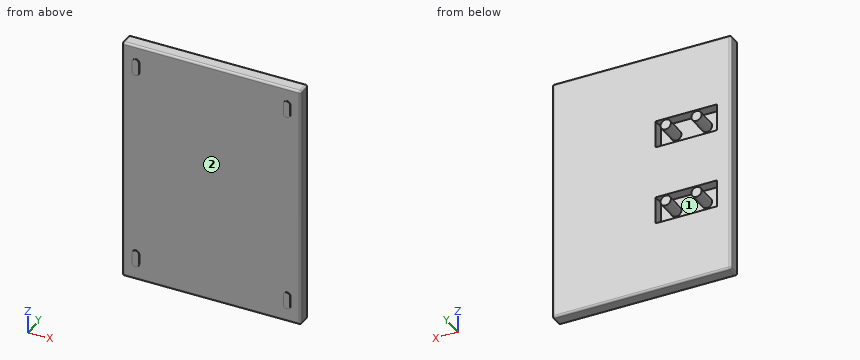
Autodesk Inventor part; units mm, degrees
ref_plane "YZ Plane" through (0, 0, 0) normal (1, 0, 0) x (0, 1, 0)
ref_plane "XZ Plane" through (0, 0, 0) normal (0, 1, 0) x (-1, 0, 0)
ref_plane "XY Plane" through (0, 0, 0) normal (0, 0, 1) x (1, 0, 0)
sketch "Sketch1" plane through (0, 0, 0) normal (0, 1, 0) x (-1, 0, 0)
  line L0 (0, 0) -> (260, 0)
  line L1 (260, 0) -> (260, -360)
  line L2 (260, -360) -> (0, -360)
  line L3 (0, -360) -> (0, 0)
  line L4 (240, -101.4) -> (150.6, -101.4)
  line L5 (150.6, -101.4) -> (150.6, -141.4)
  line L6 (150.6, -141.4) -> (240, -141.4)
  line L7 (240, -141.4) -> (240, -101.4)
  line L8 (240, -218.6) -> (150.6, -218.6)
  line L9 (150.6, -218.6) -> (150.6, -258.6)
  line L10 (150.6, -258.6) -> (240, -258.6)
  line L11 (240, -258.6) -> (240, -218.6)
  circle A0 centre (217.65, -121.4) radius 7.5
  circle A1 centre (172.95, -121.4) radius 7.5
  circle A2 centre (217.65, -238.6) radius 7.5
  circle A3 centre (172.95, -238.6) radius 7.5
  point P0 (240, -121.4)
  point P1 (150.6, -238.6)
  point P2 (240, -238.6)
  dimension "d0" = 260
  dimension "d1" = 360
  dimension "d2" = 89.4
  dimension "d3" = 40
  dimension "d4" = 89.4
  dimension "d5" = 40
  dimension "d8" = 15
  dimension "d9" = 15
  dimension "d11" = 22.35
  dimension "d12" = 15
  dimension "d13" = 15
  dimension "d14" = 22.35
  dimension "d15" = 22.35
  dimension "d16" = 22.35
  dimension "d17" = 20
  dimension "d61" = 117.2
  dimension "d62" = 101.4
  dimension "d63" = 101.4
extrude "Extrusion1" add sketch "Sketch1" along normal blind 20 contours L0 L1 L2 L3
extrude "Extrusion2" add sketch "Sketch1" along normal blind 5 contours L7 L6 L5 L4 | L11 L10 L9 L8
extrude "Extrusion3" add sketch "Sketch1" along normal blind 35 contours A0 | A1 | A2 | A3
sketch "Sketch2" plane through (0, 20, 0) normal (0, 1, 0) x (1, 0, 0)
  point P0 (0, 0)
sketch "Sketch4" plane through (0, 0, 0) normal (0, -1, 0) x (1, 0, 0)
  line L0 (-240, -335) -> (-240, -320) construction
  line L1 (-235, -335) -> (-235, -320)
  line L2 (-245, -320) -> (-245, -335)
  arc A0 (-245, -335) -> (-235, -335) centre (-240, -335) ccw
  arc A1 (-235, -320) -> (-245, -320) centre (-240, -320) ccw
  line L3 (-260, -360) -> (-260, 0)
  line L4 (0, -360) -> (-260, -360)
  line L5 (-240, -40) -> (-240, -25) construction
  line L6 (-235, -40) -> (-235, -25)
  line L7 (-245, -25) -> (-245, -40)
  arc A2 (-245, -40) -> (-235, -40) centre (-240, -40) ccw
  arc A3 (-235, -25) -> (-245, -25) centre (-240, -25) ccw
  line L8 (-20, -40) -> (-20, -25) construction
  line L9 (-15, -40) -> (-15, -25)
  line L10 (-25, -25) -> (-25, -40)
  arc A4 (-25, -40) -> (-15, -40) centre (-20, -40) ccw
  arc A5 (-15, -25) -> (-25, -25) centre (-20, -25) ccw
  line L11 (-20, -335) -> (-20, -320) construction
  line L12 (-15, -335) -> (-15, -320)
  line L13 (-25, -320) -> (-25, -335)
  arc A6 (-25, -335) -> (-15, -335) centre (-20, -335) ccw
  arc A7 (-15, -320) -> (-25, -320) centre (-20, -320) ccw
  line L14 (0, 0) -> (0, -360)
  line L15 (-260, 0) -> (0, 0)
  point P0 (-240, -327.5)
  point P1 (-240, -340)
  point P2 (-240, -32.5)
  point P3 (-240, -45)
  point P4 (-20, -32.5)
  point P5 (-20, -45)
  point P6 (-20, -327.5)
  point P7 (-20, -340)
  point P8 (-20, -20)
  point P9 (-240, -20)
  dimension "d39" = 15
  dimension "d40" = 10
  dimension "d41" = 20
  dimension "d42" = 20
  dimension "d43" = 15
  dimension "d44" = 10
  dimension "d45" = 15
  dimension "d46" = 10
  dimension "d47" = 15
  dimension "d48" = 10
  dimension "d49" = 20
  dimension "d50" = 20
  dimension "d51" = 20
  dimension "d52" = 20
  dimension "d53" = 20
  dimension "d54" = 20
extrude "Extrusion5" add sketch "Sketch4" along normal blind 1 contours A0 L2 A1 L1 | A2 L7 A3 L6 | A4 L10 A5 L9 | A6 L13 A7 L12
fillet "Fillet1" radius 3 12 edges at (-260, 20, -180) (-130, 20, 0) (-260, 10, 0) (-130, 0, 0) (0, 10, 0) (0, 20, -180) (0, 0, -180) (-130, 0, -360) (-130, 20, -360) (0, 10, -360) (-260, 10, -360) (-260, 0, -180)
fillet "Fillet2" radius 1 8 edges at (-240, 12.5, -258.6) (-240, 12.5, -218.6) (-150.6, 12.5, -218.6) (-150.6, 12.5, -258.6) (-240, 12.5, -141.4) (-150.6, 12.5, -141.4) (-150.6, 12.5, -101.4) (-240, 12.5, -101.4)
properties part number "base2"
Geometry check sheet. Reference: the model listing, model coordinates, mm. Face numbers are marked on the shaded views. A direction names the side the tool comes from. Give positions to 0.01 mm unless a question says otherwise; leave off trailing zeros. Write each loop counter-clockwise with the first axis right and the second up, starting at its lowest first coordinate (ties: lowest second). Pieces come first, ordered by that corner, then holes. Notation, with made-up numbers: M 41.25,-18.75 L 62.25,-18.75 A9 cw 62.25,-12.75 Z; hole C 17.25,45.5 d8. An arc over 180 degrees is marked long. Answer as CSV lines item,"result". Start each with the question number.
Q1. Section check D-D, the plane x = -172.95. Record the cut outline in (y, z), then the cut area to 3 significant figures.
Q2. Tool access check on the marked faces 1 and 2. Record the directions out of +Z, -Z, +X, -X, +Y, -Y that give a thin tool (end or side, any length) a straight path to the whole face; none if there is none.
Q3. Section check C-C, the plane z = -238.6. Record the cut outline in (x, y).
Q4. Section check A-A, the plane y = 12. Record the cut outline in (x, z), then the cut area to 3 significant figures.
Q5. Section check B-B, the plane x = -20. Record the cut outline in (y, z).
Q6. Material ranges on L1, parallel to Z at x = -233.5, y = 15; L2, parallel to X at y = 7.5, z = -112; L3, parallel to Z at x = -190.5, y = 19, recorded low to high.
Q7. Go/stop test with flat-tipped pins: pin 1 (20 mm diameter, centred on x = -192, z = -248.5, fed in from +Y); pin 2 (2 mm diameter, centred on y = 22, z = -127, fed in from -X); pin 3 (12 mm diameter, centred on y = 24, z = -272.5, fed in from -X). Record where each tip stops, or that it passes through.
Geometry says:
1,outline,"M 0,-357 A3 ccw 3,-360 L 17,-360 A3 ccw 20,-357 L 20,-258.6 L 5,-258.6 L 5,-246.1 L 35,-246.1 L 35,-231.1 L 5,-231.1 L 5,-218.6 L 20,-218.6 L 20,-141.4 L 5,-141.4 L 5,-128.9 L 35,-128.9 L 35,-113.9 L 5,-113.9 L 5,-101.4 L 20,-101.4 L 20,-3 A3 ccw 17,0 L 3,0 A3 ccw 0,-3 Z"
1,area,"6,890 mm^2"
2,face 1,"+Y"
2,face 2,"-Y"
3,outline,"M -260,3 A3 ccw -257,0 L -3,0 A3 ccw 0,3 L 0,17 A3 ccw -3,20 L -150.6,20 L -150.6,5 L -165.45,5 L -165.45,35 L -180.45,35 L -180.45,5 L -210.15,5 L -210.15,35 L -225.15,35 L -225.15,5 L -240,5 L -240,20 L -257,20 A3 ccw -260,17 Z"
4,outline,"M -260,-357 A3 ccw -257,-360 L -3,-360 A3 ccw 0,-357 L 0,-3 A3 ccw -3,0 L -257,0 A3 ccw -260,-3 Z; C -217.65,-238.6 d15; C -217.65,-121.4 d15; C -172.95,-238.6 d15; C -172.95,-121.4 d15; hole M -240,-257.6 A1 ccw -239,-258.6 L -151.6,-258.6 A1 ccw -150.6,-257.6 L -150.6,-219.6 A1 ccw -151.6,-218.6 L -239,-218.6 A1 ccw -240,-219.6 Z; hole M -240,-140.4 A1 ccw -239,-141.4 L -151.6,-141.4 A1 ccw -150.6,-140.4 L -150.6,-102.4 A1 ccw -151.6,-101.4 L -239,-101.4 A1 ccw -240,-102.4 Z"
4,area,"87,100 mm^2"
5,outline,"M -1,-340 L 0,-340 L 0,-357 A3 ccw 3,-360 L 17,-360 A3 ccw 20,-357 L 20,-3 A3 ccw 17,0 L 3,0 A3 ccw 0,-3 L 0,-20 L -1,-20 L -1,-45 L 0,-45 L 0,-315 L -1,-315 Z"
6,L1,"-360 to -258.6, -218.6 to -141.4, -101.4 to 0"
6,L2,"-260 to -240, -150.6 to 0"
6,L3,"-359.24 to -258.6, -218.6 to -141.4, -101.4 to -0.76"
7,pin 1,"y = 5"
7,pin 2,"x = -223.57"
7,pin 3,"x = -259.83"
